from build123d import *

# Parameters (mm, degrees)
SKETCH_W        = 370
SKETCH_H        = 20
PAD_DEPTH       = 20
SKETCH001_R     = 4.75
POCKET_DEPTH    = 5
SKETCH002_R     = 2.75
POCKET001_DEPTH = 15


with BuildPart() as part:
    # Sketch → Pad (new body)
    with BuildSketch(Plane.XY):
        Rectangle(SKETCH_W, SKETCH_H)
    extrude(amount=-PAD_DEPTH)

    # Sketch001 (on Face5 of Pad) → Pocket (cut)
    with BuildSketch(Plane.XY):
        with Locations((168, 0)):
            Circle(SKETCH001_R)
        with Locations((-168, 0)):
            Circle(SKETCH001_R)
    extrude(amount=-POCKET_DEPTH, mode=Mode.SUBTRACT)

    # Sketch002 (on Face4 of Pocket) → Pocket001 (cut)
    with BuildSketch(Plane.XY):
        with Locations((-168, 0)):
            Circle(SKETCH002_R)
        with Locations((168, 0)):
            Circle(SKETCH002_R)
    extrude(amount=-POCKET001_DEPTH, mode=Mode.SUBTRACT)


solid = part.part
Design review of the part built by this model. Coordinates are the model's own, in mm. A direction names the side the tool comes from. Give positions to 0.01 mm unless a question says otherwise; leave off trailing zeros. Return JSON: item names as keys, results as strings. Group by question number.
Item 1: The part is to be moulded in two halves that separate along Y. For faces 3 (the flat face through (-3, 0, -20)), 4 (the flat face through (-3, 10, -10)), 5 (the cylindrical face through (172.388, -1.819, -2.465)), say which applies: pulls with the +Y half, pulls with the -Y half, needs draft (parallel to the pull), parting line crosses it, or undercut.
Item 2: Clearance check with flat-ended pins moving along their axes: pin 1 Ø3 at (x, y) = (-170.5, -1) entering from +Z; pin 2 Ø3.5 at (x, y) = (-168, 0) entering from +Z. State where each tip first meets the part, or that it passes through.
Item 3: Wall thickness on line 1 along Y through (x, z) = (-168, -1); line 2 along X through (y, z) = (-3.75, -3.25); line 3 along X through (y, z) = (-1.5, -8): over which ranges is each line inside the solid? List them lowest first.
Item 4: Tool access review of faces 1 (the flat face through (185, 0, -10)), 2 (the flat face through (171, 0, -5)): name each direction out of +Z, -Z, +X, -X, +Y, -Y from which nothing blocks a thin tool from reaching the whole face with its end or side.
Return value:
{
 "1": {"face 3": "needs draft", "face 4": "pulls with the +Y half", "face 5": "undercut"},
 "2": {"pin 1": "stops at z = -5", "pin 2": "stops at z = -15"},
 "3": {"line 1": "y = -10 to -4.75, 4.75 to 10", "line 2": "x = -185 to -170.92, -165.08 to 165.08, 170.92 to 185", "line 3": "x = -185 to -170.3, -165.7 to 165.7, 170.3 to 185"},
 "4": {"face 1": "+Z, -Z, +X, +Y, -Y", "face 2": "+Z"}
}
